Autodesk Inventor part; units mm, degrees
ref_plane "YZ Plane" through (0, 0, 0) normal (1, 0, 0) x (0, 1, 0)
ref_plane "XZ Plane" through (0, 0, 0) normal (0, 1, 0) x (-1, 0, 0)
ref_plane "XY Plane" through (0, 0, 0) normal (0, 0, 1) x (1, 0, 0)
sketch "Sketch1" plane through (0, 0, 0) normal (0, 1, 0) x (-1, 0, 0)
  circle A0 centre (0, 0) radius 3.175 construction
  line L0 (3.556, 12.7) -> (-6.604, 12.7)
  line L1 (-6.604, 12.7) -> (-6.604, -12.7)
  line L2 (-6.604, -12.7) -> (3.556, -12.7)
  line L3 (3.556, -12.7) -> (3.556, 12.7)
  line L4 (5.588, 0) -> (-8.636, 0)
  dimension "d0" = 6.35
  dimension "d1" = 3.556
  dimension "d2" = 10.16
  dimension "d3" = 25.4
extrude "Extrusion1" add sketch "Sketch1" along normal blind 3.175
sketch "Sketch2" plane through (0, 3.175, 0) normal (0, 1, 0) x (1, 0, 0)
  line L0 (-5.588, 0) -> (8.636, 0)
  line L1 (0, 17.78) -> (0, -17.78)
  circle A0 centre (0, 0) radius 3.2004
  dimension "d6" = 6.4008
extrude "Extrusion2" cut sketch "Sketch2" against normal blind 2.3813
sketch "Sketch3" plane through (0, 0, 0) normal (0, -1, 0) x (1, 0, 0)
  line L0 (0, -17.78) -> (0, 17.78)
  line L1 (-5.588, 0) -> (8.636, 0)
  point P0 (0, 0)
  point P1 (0, 5.715)
  point P2 (0, -5.715)
  dimension "d9" = 11.43
hole "Hole1" at (0, 0, 5.715) at (0, 0, -5.715) direction (0, 1, 0) diameter 2.4384 depth 25.4 tip angle 118 countersink diameter 4.3688 countersink angle 82
chamfer "Chamfer3" distance 3.175 angle 45 1 edges at (6.604, 0, 0)
sketch "Sketch4" plane through (0, 3.175, 0) normal (0, 1, 0) x (1, 0, 0)
  arc A0 (-3.6703, 0) -> (-7.9936, 12.7) centre (-24.4856, 0) ccw
  line L0 (-55.6819, 0) -> (16.985, 0)
  line L1 (-3.556, -12.7) -> (6.604, -12.7)
  line L2 (6.604, 12.7) -> (-3.556, 12.7)
  line L3 (-3.556, 12.7) -> (-3.556, -12.7)
  line L4 (-3.556, -12.7) -> (-7.9936, -12.7)
  line L5 (-3.556, 12.7) -> (-7.9936, 12.7)
  line L6 (-3.556, -12.7) -> (-3.556, 12.7)
  arc A1 (-7.9936, -12.7) -> (-3.6703, 0) centre (-24.4856, 0) ccw
  arc A2 (-7.9936, 12.7) -> (-7.9936, -12.7) centre (-24.4856, 0) ccw construction
  point P0 (0, 0)
  dimension "d26" = 24.4856
  dimension "d27" = 41.6306
extrude "Extrusion3" add sketch "Sketch4" against normal blind 3.175
chamfer "Chamfer4" distance 3.175 angle 45 2 edges at (-2.282, 0, 12.7) (-2.282, 0, -12.7)
chamfer "Chamfer5" distance 0.508 angle 45 1 edges at (-3.6703, 0, 0)
sketch "Sketch5" plane through (0, 3.175, 0) normal (0, 1, 0) x (1, 0, 0)
  line L0 (-6.096, -13.97) -> (-6.096, 13.97)
  line L1 (6.604, -12.7) -> (6.604, 12.7)
  line L2 (-6.096, -13.97) -> (-12.446, -13.97)
  line L3 (-12.446, -13.97) -> (-12.446, 13.97)
  line L4 (-12.446, 13.97) -> (-6.096, 13.97)
  circle A0 centre (0, 0) radius 3.2004
  line L5 (-16.256, 0) -> (10.414, 0)
  dimension "d36" = 12.7
  dimension "d37" = 6.35
  dimension "d38" = 27.94
extrude "Extrusion4" cut sketch "Sketch5" against normal blind 3.175 contours L2 L3 L5 L0 | L5 L3 L4 L0
sketch "Sketch6" plane through (0, 0, 0) normal (0, -1, 0) x (1, 0, 0)
  circle A0 centre (0, 0) radius 3.2004
  line L0 (-5.588, 0) -> (8.636, 0)
  line L1 (0, -17.78) -> (0, 17.78)
  line L2 (0, 0) -> (2.4318, -2.8981) construction
  line L3 (-3.006, 2.3476) -> (1.79, -3.368)
  line L4 (2.3491, -3.417) -> (2.9571, -2.9067)
  line L5 (3.006, -2.3476) -> (-1.79, 3.368)
  line L6 (-2.3491, 3.417) -> (-2.9571, 2.9067)
  line L7 (-3.2612, 2.6516) -> (3.2612, -2.6516) construction
  line L8 (2.0451, -3.6721) -> (-2.0451, 3.6721) construction
  arc A1 (2.9571, -2.9067) -> (3.006, -2.3476) centre (2.702, -2.6027) ccw
  arc A2 (1.79, -3.368) -> (2.3491, -3.417) centre (2.094, -3.1129) ccw
  arc A3 (-2.9571, 2.9067) -> (-3.006, 2.3476) centre (-2.702, 2.6027) ccw
  arc A4 (-1.79, 3.368) -> (-2.3491, 3.417) centre (-2.094, 3.1129) ccw
  dimension "d41" = 50
  dimension "d42" = 8.255
  dimension "d43" = 1.5875
  dimension "d46" = 0.3969
  dimension "d47" = 140
extrude "Extrusion5" [suppressed]
equation "\"d4\" = bearing_thickness"
equation "\"d28\" = bearing_thickness"
equation "\"d39\" = bearing_thickness"
properties part number "bearing_insert_thick_flat_projecting" material "Stainless Steel, 440C"
Input: part model. Units: mm. Frame: model coordinates. A direction names the side the tool comes from. Coordinates: 2 decimals unless noted, no trailing zeros. Order: outer loops, then holes, each group sorted by start corner. A loop starts at its lowest first (then second) coordinate and runs counter-clockwise, first axis right, second up. Notation, with made-up numbers: M 42.5,36 L 50.5,36 A22 ccw 50.5,54 Z; hole C 17,50 d5. An arc over 180 degrees is marked long. Answer in a Markdown table with one row per item.
(1) Access query for faces 1 (the cylindrical face through (-4.303, 1.86, 5.093)), 2 (the flat face through (0, 0, 0)), 3 (the flat face through (0, 0.794, 0)). Directions: +Z, -Z, +X, -X, +Y, -Y. A direction counts if a zero-diameter tool reaches every point of the face in a straight line with its end or side. Return the directions, or none.
Numbers:
| item | result |
|---|---|
| face 1 | -X, +Y, -Y |
| face 2 | +Z, -Z, +X, -X, -Y |
| face 3 | +Y |
(2) Section query B-B, the plane y = 2. Output: boundary loops of the cut face in (x, z) (1 decimal), plus the area to 3 significant figures.
Numbers:
| item | result |
|---|---|
| outline | M -6.1,-11.5 L 5.4,-11.5 L 5.4,11.5 L -6.1,11.5 L -6.1,9.8 A20.8 cw -3.7,0 A20.8 cw -6.1,-9.8 Z; hole C 0,0 d6.4; hole C 0,-5.7 d2.4; hole C 0,5.7 d2.4 |
| area | 192 mm^2 |
(3) Draft query along Z for faces 4 (the cylindrical face through (-4.27, 1.86, -4.96)), 5 (the flat face through (-6.096, 2, -11)), 6 (the cylindrical face through (-2.54, 2, 1.95)), 7 (the flat face through (-1.068, 1.609, -11.135)). Return one class per face: pulls with the +Z half, pulls with the -Z half, needs draft (parallel to the pull), parting line crosses it, or undercut.
Numbers:
| item | result |
|---|---|
| face 4 | undercut |
| face 5 | needs draft |
| face 6 | undercut |
| face 7 | pulls with the -Z half |
(4) Material intervals for line 1 (Z direction, x = 0.75, y = 2.35); line 2 (Z direction, x = 0, y = 1.7); line 3 (Y direction, x = 0.75, z = -2.75), sorted ascending. Write a range as [from, to].
Numbers:
| item | result |
|---|---|
| line 1 | z = [-11.88, -6.68], [-4.75, -3.11], [3.11, 4.75], [6.68, 11.88] |
| line 2 | z = [-11.23, -6.93], [-4.5, -3.2], [3.2, 4.5], [6.93, 11.23] |
| line 3 | y = [0, 0.79] |
(5) Section query A-A, the plane x = 0. Give the number of separate pieces and of enclosed holes in the cut face, plus the area to 3 significant figures.
Numbers:
| item | result |
|---|---|
| separate pieces | 3 |
| enclosed holes | 0 |
| area | 37.7 mm^2 |
(6) Contact query for flat-ended pins moving along their axis: pin 1 Ø1 at (y, z) = (1.5, -7) entering from +X; pin 2 Ø1.5 at (x, z) = (0, -5.715) entering from +Y; pin 3 Ø4 at (x, z) = (0, 0) entering from -Y; pin 4 Ø1.9 at (x, z) = (0.5, 1) entering from +Y. Output: stop coordinate, or through.
Numbers:
| item | result |
|---|---|
| pin 1 | stops at x = 5.43 |
| pin 2 | passes through |
| pin 3 | stops at y = 0 |
| pin 4 | stops at y = 0.79 |
